```python
from build123d import *

# Parameters (mm, degrees)
SKETCH1_W           = 21.9075
SKETCH1_H           = 15.875
BOSS_EXTRUDE1_DEPTH = 101.6
FILLET1_R           = 1.5875
SKETCH2_R           = 2.3114
CUT_EXTRUDE2_DEPTH  = 21.9075
CUT_EXTRUDE3_REACH  = 107.14
SKETCH4_W           = 21.9075
SKETCH4_H           = 15.875
CUT_EXTRUDE4_DEPTH  = 12.7


with BuildPart() as part:
    # Sketch1 → Boss-Extrude1 (new body)
    with BuildSketch(Plane.XY):
        with Locations((10.95375, 7.9375)):
            Rectangle(SKETCH1_W, SKETCH1_H)
    extrude(amount=BOSS_EXTRUDE1_DEPTH)

    # Fillet1
    fillet1_edges = [part.edges().sort_by_distance(p)[0] for p in [
        (0, 15.875, 50.8),
        (21.9075, 15.875, 50.8),
    ]]
    fillet(fillet1_edges, radius=FILLET1_R)

    # Sketch2 → Cut-Extrude2 (cut)
    with BuildSketch(Plane(origin=(21.9075, 0, 0), x_dir=(0, 0, -1), z_dir=(1, 0, 0))):
        with Locations((-57.15, 9.8298)):
            Circle(SKETCH2_R)
        with Locations((-44.45, 9.8298)):
            Circle(SKETCH2_R)
        with Locations((-82.55, 9.8298)):
            Circle(SKETCH2_R)
        with Locations((-6.35, 9.8298)):
            Circle(SKETCH2_R)
        with Locations((-19.05, 9.8298)):
            Circle(SKETCH2_R)
    extrude(amount=-CUT_EXTRUDE2_DEPTH, mode=Mode.SUBTRACT)

    # Sketch3 → Cut-Extrude3 (cut, up to next)
    with BuildSketch(Plane.XZ, mode=Mode.PRIVATE) as cut_extrude3_sk1:
        Polygon((19.246822331, 98.58883), (15.360677669, 98.58883), (13.417605338, 95.22333), (15.360677669, 91.85783), (19.246822331, 91.85783), (21.189894662, 95.22333), align=None)
    cut_extrude3_tool1 = extrude(cut_extrude3_sk1.sketch, amount=-CUT_EXTRUDE3_REACH, mode=Mode.PRIVATE) & part.part
    # Sketch3 → Cut-Extrude3 (cut, up to next)
    with BuildSketch(Plane.XZ, mode=Mode.PRIVATE) as cut_extrude3_sk2:
        Polygon((12.896822331, 28.7655), (9.010677669, 28.7655), (7.067605338, 25.4), (9.010677669, 22.0345), (12.896822331, 22.0345), (14.839894662, 25.4), align=None)
    cut_extrude3_tool2 = extrude(cut_extrude3_sk2.sketch, amount=-CUT_EXTRUDE3_REACH, mode=Mode.PRIVATE) & part.part
    add(cut_extrude3_tool1.solids().sort_by_distance((17.30375, 0, 95.22333))[0], mode=Mode.SUBTRACT)
    add(cut_extrude3_tool2.solids().sort_by_distance((10.95375, 0, 25.4))[0], mode=Mode.SUBTRACT)

    # Sketch4 → Cut-Extrude4 (cut)
    with BuildSketch(Plane(origin=(0, 0, 0), x_dir=(-1, 0, 0), z_dir=(0, 0, -1))):
        with Locations((-10.95375, 7.9375)):
            Rectangle(SKETCH4_W, SKETCH4_H)
    extrude(amount=-CUT_EXTRUDE4_DEPTH, mode=Mode.SUBTRACT)


solid = part.part
```
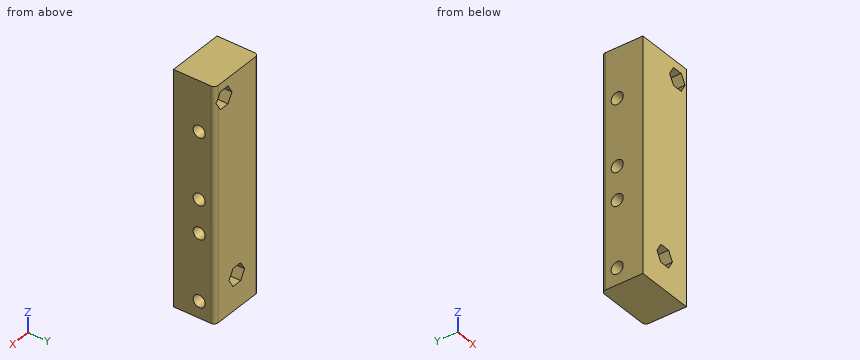
Model file for the job. Use its own axes, mm. Coordinates: 2 decimals unless noted, no trailing zeros. Loops run counter-clockwise (first coordinate to the right, second up) from the corner with the lowest first, then second, coordinate; pieces in that order, holes last. Notation, with made-up numbers: (-0.75, -3.75) - (12.25, -3.75) arc R31 cw to (12.25, 35.25) - close; hole circle Ø7 at (86, 77.25). An arc over 180 degrees is marked (long way). Answer as a JSON object with one key per item and string values. Group by question number.
(1) Cut at C-C (y = 6). Give the cut face in (x, z), then the cut area to 3 significant figures.
(2) Flat gauge pin, fed straight in: pin 1 (3.5 mm diameter, centred on y = 9.83, z = 19.05, fed in from -X). Where does the tip first touch, or does it go through?
(3) Cut at A-A (x = 18). Give the cut face in (y, z) (3 decimals).
(4) Probe line 1 along Z through (x, y) = (9, 5.5); line 2 along Y through (x, z) = (12.25, 19.05) (3 decimals); line 3 along Z through (x, y) = (16.5, 13). List the from-to ranges inside material, lowest first.
(5) Cut at B-B (z = 44.45). Give the cut face in (x, y) (1 decimal).
(6) Cut at D-D (x = 5.5). Give the cut face in (y, z) (3 decimals).
Geometry says:
{
 "1": {"outline": "(0, 12.7) - (21.91, 12.7) - (21.91, 101.6) - (0, 101.6) - close; hole (7.07, 25.4) - (9.01, 22.03) - (12.9, 22.03) - (14.84, 25.4) - (12.9, 28.77) - (9.01, 28.77) - close; hole (13.42, 95.22) - (15.36, 91.86) - (19.25, 91.86) - (21.19, 95.22) - (19.25, 98.59) - (15.36, 98.59) - close", "area": "1,870 mm^2"},
 "2": {"pin 1": "passes through"},
 "3": {"outline": "(0, 12.7) - (15.875, 12.7) - (15.875, 91.858) - (0, 91.858) - close; (0, 98.589) - (15.875, 98.589) - (15.875, 101.6) - (0, 101.6) - close; hole circle Ø4.623 at (9.83, 19.05); hole circle Ø4.623 at (9.83, 44.45); hole circle Ø4.623 at (9.83, 57.15); hole circle Ø4.623 at (9.83, 82.55)"},
 "4": {"line 1": "z = 12.7 to 22.05, 28.75 to 101.6", "line 2": "y = 0 to 7.518, 12.141 to 15.875", "line 3": "z = 12.7 to 91.86, 98.59 to 101.6"},
 "5": {"outline": "(0, 0) - (21.9, 0) - (21.9, 7.5) - (0, 7.5) - close; (0, 12.1) - (21.9, 12.1) - (21.9, 14.3) arc R1.6 ccw to (20.3, 15.9) - (1.6, 15.9) arc R1.6 ccw to (0, 14.3) - close"},
 "6": {"outline": "(0, 12.7) - (15.875, 12.7) - (15.875, 101.6) - (0, 101.6) - close; hole circle Ø4.623 at (9.83, 19.05); hole circle Ø4.623 at (9.83, 44.45); hole circle Ø4.623 at (9.83, 57.15); hole circle Ø4.623 at (9.83, 82.55)"}
}
